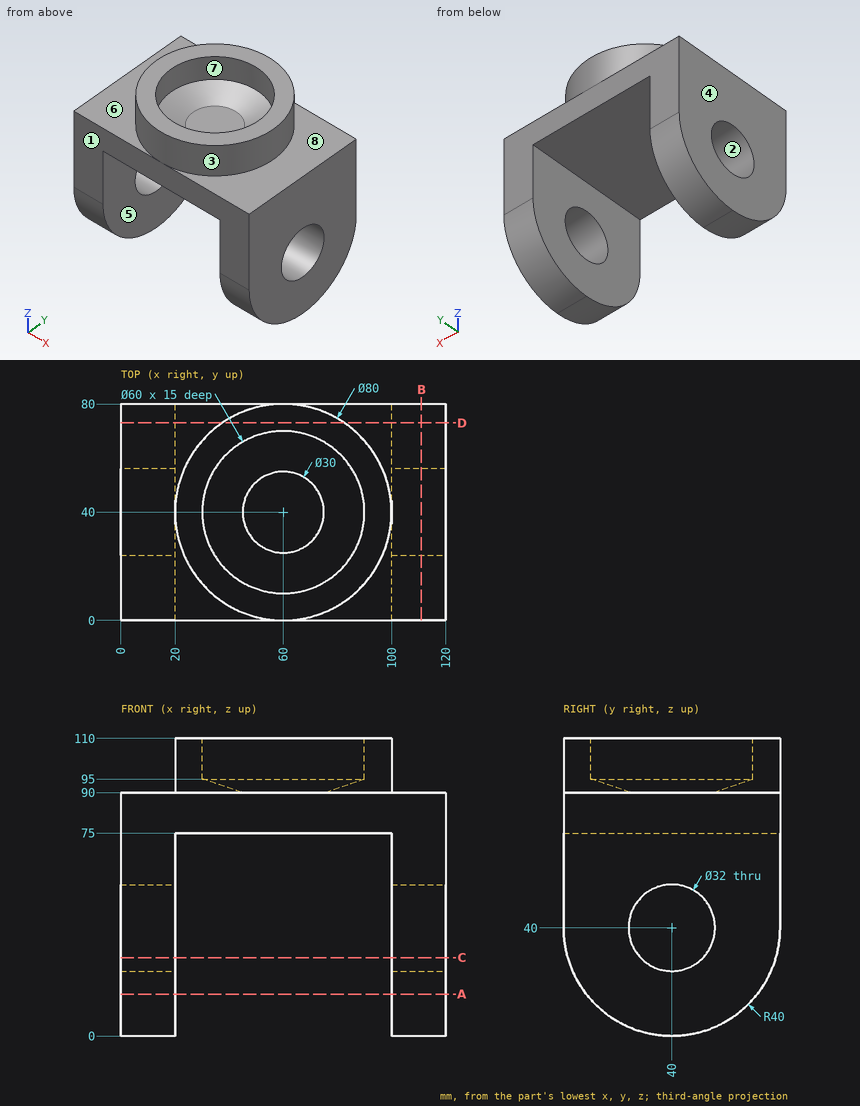
Input: dimensioned drawing with shaded views. Units: mm. Origin: part minimum x, y, z. A direction names the side the tool comes from. Give positions to 0.01 mm unless a question says otherwise; leave off trailing zeros. Loops run counter-clockwise (first coordinate to the right, second up) from the corner with the lowest first, then second, coordinate; pieces in that order, holes last. Notation, with made-up numbers: M -25.5,36.5 L 12.5,36.5 A7 ccw 12.5,40.5 Z; hole C 4,16.25 d6. An arc over 180 degrees is marked long. Put each result on its own line as item: value. Start each with the question number.
1) Pull-direction query (Y, two-part tool) for the marked faces 1, 2 and 3; classes: pulls with the +Y half, pulls with the -Y half, needs draft (parallel to the pull), parting line crosses it, or undercut.
2) Cut plane D-D (y = 73). Output: boundary loops of the cut face in (x, z), then the cut area to 3 significant figures.
3) Ray query, line 1 along X through (y, z) = (42.5, 24); line 2 along Z through (x, y) = (93.5, 18); line 3 along X through (y, z) = (63, 102.5). Return the intervals inside material, ascending.
4) Cut plane A-A (z = 15.5). Output: boundary loops of the cut face in (x, y), then the cut area to 3 significant figures.
5) Cut plane B-B (x = 111). Output: boundary loops of the cut face in (y, z).
6) Contact query for flat-ended pins moving along their axis: pin 1 (24 mm diameter, centred on x = 67.5, y = 42.5, fed in from -Z); pin 2 (5 mm diameter, centred on x = 107.5, z = 15.5, fed in from +Y); pin 3 (3 mm diameter, centred on x = 75.5, y = 24, fed in from +Z). Output: stop coordinate, or through.
7) Access query for the marked faces 4, 5, 6, 7 and 8. Directions: +Z, -Z, +X, -X, +Y, -Y. A direction counts if a zero-diameter tool reaches every point of the face in a straight line with its end or side. Return the directions, or none.
8) Cut plane C-C (z = 29). Output: boundary loops of the cut face in (x, y).
Verdict:
1. face 1: pulls with the -Y half
1. face 2: undercut
1. face 3: parting line crosses it
2. outline: M 0,17.39 L 20,17.39 L 20,75 L 100,75 L 100,17.39 L 120,17.39 L 120,90 L 82.61,90 L 82.61,110 L 37.39,110 L 37.39,90 L 0,90 Z
2. area: 5,010 mm2
3. line 1: 0 to 20, 100 to 120
3. line 2: 75 to 90
3. line 3: 27.27 to 40.74, 79.26 to 92.73
4. outline: M 0,8.38 L 20,8.38 L 20,71.62 L 0,71.62 Z; M 100,8.38 L 120,8.38 L 120,71.62 L 100,71.62 Z
4. area: 2,530 mm2
5. outline: M 0,40 A40 ccw 40,0 A40 ccw 80,40 L 80,90 L 0,90 Z; hole C 40,40 d32
6. pin 1: z = 75
6. pin 2: y = 73.41
6. pin 3: z = 92.93
7. face 4: +Z, -Z, -X, +Y, -Y
7. face 5: -Z, +Y, -Y
7. face 6: +Z, -X
7. face 7: +Z
7. face 8: +Z, +X
8. outline: M 0,1.54 L 20,1.54 L 20,28.38 L 0,28.38 Z; M 0,51.62 L 20,51.62 L 20,78.46 L 0,78.46 Z; M 100,1.54 L 120,1.54 L 120,28.38 L 100,28.38 Z; M 100,51.62 L 120,51.62 L 120,78.46 L 100,78.46 Z
